```python
from build123d import *

# Parameters (mm, degrees)
F0_W      = 50.8
F0_H      = 38.1
F1_DEPTH  = 31.75
F3_DEPTH  = 31.75
F5_DEPTH  = 31.75
F7_DEPTH  = 19.05
F9_DEPTH  = 19.05
F11_DEPTH = 12.7
F13_DEPTH = 12.7


with BuildPart() as f1:
    # F0 (on Front) → F1 (new body)
    with BuildSketch(Plane.XZ):
        with Locations((25.4, 19.05)):
            Rectangle(F0_W, F0_H)
    extrude(amount=F1_DEPTH)

    # F2 (on face) → F3 (cut)
    with BuildSketch(Plane.XZ.offset(31.75)):
        Polygon((50.8, 38.1), (31.75, 38.1), (50.8, 12.7), align=None)
    extrude(amount=-F3_DEPTH, mode=Mode.SUBTRACT)

    # F4 (on face) → F5 (cut)
    with BuildSketch(Plane.XZ.offset(31.75)):
        Polygon((0, 12.7), (19.05, 38.1), (0, 38.1), align=None)
    extrude(amount=-F5_DEPTH, mode=Mode.SUBTRACT)

    # F6 (on face) → F7 (cut)
    with BuildSketch(Plane.XZ.offset(31.75)):
        Polygon((31.75, 12.7), (50.8, 12.7), (31.75, 38.1), align=None)
    extrude(amount=-F7_DEPTH, mode=Mode.SUBTRACT)

    # F8 (on face) → F9 (cut)
    with BuildSketch(Plane.XZ.offset(31.75)):
        Polygon((19.05, 38.1), (0, 12.7), (19.05, 12.7), align=None)
    extrude(amount=-F9_DEPTH, mode=Mode.SUBTRACT)

    # F10 (on face) → F11 (join)
    with BuildSketch(Plane(origin=(0, 0, 0), x_dir=(-1, 0, 0), z_dir=(0, 1, 0))):
        Polygon((0, 38.1), (-19.05, 38.1), (0, 12.7), align=None)
    extrude(amount=-F11_DEPTH)

    # F12 (on face) → F13 (cut)
    with BuildSketch(Plane(origin=(19.05, 0, 0), x_dir=(0, -1, 0), z_dir=(-1, 0, 0))):
        Polygon((31.75, 38.1), (12.7, 38.1), (31.75, 12.7), align=None)
    extrude(amount=-F13_DEPTH, mode=Mode.SUBTRACT)


solid = f1.part
```
Can you work these out from the model? Positions are in its coordinate system, mm. A direction names the side the tool comes from. Coordinates: 2 decimals unless noted, no trailing zeros. Loops run counter-clockwise (first coordinate to the right, second up) from the corner with the lowest first, then second, coordinate; pieces in that order, holes last. Notation, with made-up numbers: (34.5, 51) - (70.5, 51) arc R12 cw to (70.5, 71) - close; hole circle Ø1 at (84, -36.5). An arc over 180 degrees is marked (long way). Use a Markdown table: item, result.
Item 1: I want a section at D-D on y = -5. Please give me the cut outline in (x, z).
Numbers:
| item | result |
|---|---|
| outline | (0, 0) - (50.8, 0) - (50.8, 12.7) - (31.75, 38.1) - (0, 38.1) - close |
Item 2: Will these pins go through, and if not, where does the flat tip stop? pin 1 (5.5 mm diameter, centred on y = -26.5, z = 20.5, fed in from +X); pin 2 (15 mm diameter, centred on x = 39.5, z = 23.5, fed in from -Y); pin 3 (9.5 mm diameter, centred on y = -20.5, z = 25, fed in from -X).
Numbers:
| item | result |
|---|---|
| pin 1 | stops at x = 31.75 |
| pin 2 | stops at y = -12.7 |
| pin 3 | stops at x = 19.05 |
Item 3: If I drill on probe 1 along Z at (x, y) = (48.5, -24); probe 2 along X at (y, z) = (-29.5, 13.5); probe 3 along Y at (x, z) = (19, 13), over which ranges is the centre line in solid material (lowest first)? Write a range as from..to.
Numbers:
| item | result |
|---|---|
| probe 1 | z = 0..12.7 |
| probe 2 | x = 19.05..31.75 |
| probe 3 | y = -12.7..0 |
Item 4: For faces 1 (the face through (19.05, -18, 20)), 2 (the face through (37, -12.7, 20)), 3 (the face through (50.8, -16, 6)), which set-ups out of +Z, -Z, +X, -X, +Y, -Y let a thin tool reach every point of the face, with its end or its side?
Numbers:
| item | result |
|---|---|
| face 1 | +Z, -X, -Y |
| face 2 | +Z, +X, -Y |
| face 3 | +Z, -Z, +X, +Y, -Y |
Item 5: I want a section at C-C on z = 14. Please give me the cut outline in (x, y) (3 decimals).
Numbers:
| item | result |
|---|---|
| outline | (0, -12.7) - (19.05, -12.7) - (19.05, -30.775) - (31.75, -30.775) - (31.75, -12.7) - (49.825, -12.7) - (49.825, 0) - (0, 0) - close |
Item 6: I want a section at B-B on x = 22.5. Please give me the cut outline in (y, z), and give its area (3 significant figures).
Numbers:
| item | result |
|---|---|
| outline | (-31.75, 0) - (0, 0) - (0, 38.1) - (-12.7, 38.1) - (-31.75, 12.7) - close |
| area | 968 mm2 |
Item 7: I want a section at A-A on y = -16. Please give me the cut outline in (x, z).
Numbers:
| item | result |
|---|---|
| outline | (0, 0) - (50.8, 0) - (50.8, 12.7) - (31.75, 12.7) - (31.75, 33.7) - (19.05, 33.7) - (19.05, 12.7) - (0, 12.7) - close |
